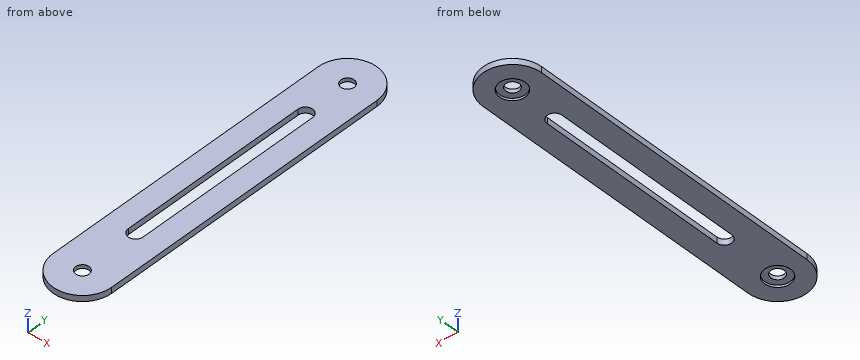
```python
from build123d import *

# Parameters (mm, degrees)
SKETCH_1_R          = 8.75
EXTRUDE_1_DEPTH     = 4
EXTRUDE_START       = -2.5
SKETCH_3_R          = 8.75
SKETCH_3_R_2        = 4.5
EXTRUDE_2_DEPTH     = 2.5
CUT_EXTRUDE_2_DEPTH = 221.943431674


with BuildPart() as part:
    # 草图1 → 凸台-拉伸1 (new body)
    with BuildSketch(Plane.XY):
        with BuildLine():
            Line((-20, 0), (-20, -200))
            ThreePointArc((-20, -200), (0, -220), (20, -200))
            Line((20, -200), (20, 0))
            ThreePointArc((20, 0), (0, 20), (-20, 0))
        make_face()
        Circle(SKETCH_1_R, mode=Mode.SUBTRACT)
        with Locations((0, -200)):
            Circle(SKETCH_1_R, mode=Mode.SUBTRACT)
    extrude(amount=EXTRUDE_1_DEPTH)

    # 草图3 → 凸台-拉伸2 (add)
    # profile 1 of 2: a face of its own
    with BuildSketch(Plane.XY.offset(4).offset(EXTRUDE_START)):
        Circle(SKETCH_3_R)
        Circle(SKETCH_3_R_2, mode=Mode.SUBTRACT)
    # profile 2 of 2: a face of its own
    with BuildSketch(Plane.XY.offset(4).offset(EXTRUDE_START)):
        with Locations((0, -200)):
            Circle(SKETCH_3_R)
        with Locations((0, -200)):
            Circle(SKETCH_3_R_2, mode=Mode.SUBTRACT)
    extrude(amount=EXTRUDE_2_DEPTH)

    # 草图2 → 切除-拉伸2 (cut, through all)
    with BuildSketch(Plane.XY.offset(4)):
        with BuildLine():
            Line((-5, -31.845004689), (-5, -159.845004689))
            ThreePointArc((-5, -159.845004689), (0, -164.845004689), (5, -159.845004689))
            Line((5, -159.845004689), (5, -31.845004689))
            ThreePointArc((5, -31.845004689), (0, -26.845004689), (-5, -31.845004689))
        make_face()
    extrude(amount=-CUT_EXTRUDE_2_DEPTH, mode=Mode.SUBTRACT)


solid = part.part
```
Geometry: final body of the model. Coordinates: model frame, mm. Round coordinates to 2 decimals unless told otherwise and drop trailing zeros. Write each loop counter-clockwise with the first axis right and the second up, starting at its lowest first coordinate (ties: lowest second). Pieces come first, ordered by that corner, then holes.
Item 1: Section query A-A (x = 0). Return loops of the section in (y, z) (3 decimals).
Item 2: Pin query (flat end, axial travel): P1, Ø2, axis at x = 6.5, z = 2, coming from the -Y side; P2, Ø5, axis at x = -0.5, y = -3.5, coming from the -Z side. Return the tip coordinate at first contact, or that it passes through.
Item 3: Section query B-B (y = -128). Return loops of the section in (x, z).
Item 4: Material intervals for L1, parallel to Y at x = 0, z = 1.2 (3 decimals); L2, parallel to Y at x = 0, z = 2.65 (3 decimals); L3, parallel to X at y = -90.5, z = 0.3, sorted ascending.
Completed:
1. outline: (-220, 0) - (-208.75, 0) - (-208.75, 1.5) - (-204.5, 1.5) - (-204.5, 4) - (-220, 4) - close; (-195.5, 1.5) - (-191.25, 1.5) - (-191.25, 0) - (-164.845, 0) - (-164.845, 4) - (-195.5, 4) - close; (-26.845, 0) - (-8.75, 0) - (-8.75, 1.5) - (-4.5, 1.5) - (-4.5, 4) - (-26.845, 4) - close; (4.5, 1.5) - (8.75, 1.5) - (8.75, 0) - (20, 0) - (20, 4) - (4.5, 4) - close
2. P1: stops at y = -219.23
2. P2: stops at z = 1.5
3. outline: (-20, 0) - (-5, 0) - (-5, 4) - (-20, 4) - close; (5, 0) - (20, 0) - (20, 4) - (5, 4) - close
4. L1: y = -220 to -208.75, -191.25 to -164.845, -26.845 to -8.75, 8.75 to 20
4. L2: y = -220 to -204.5, -195.5 to -164.845, -26.845 to -4.5, 4.5 to 20
4. L3: x = -20 to -5, 5 to 20
